For this review, take the finished solid that the model builds, in its own axes (mm). Coordinates: 2 decimals unless noted, no trailing zeros. Loops run counter-clockwise (first coordinate to the right, second up) from the corner with the lowest first, then second, coordinate; pieces in that order, holes last.
1. Take a section at A-A, the plane y = 130. State the section outline as (x, z) points, then the cut area to 3 significant figures.
2. Take a section at C-C, the plane x = -64. State the section outline as (y, z) points, then the cut area to 3 significant figures.
3. To check wall thickness, follow probe 1 along X at (y, z) = (80, 0.55); probe 2 along X at (y, z) = (145.5, 1.6); probe 3 along Y at (x, z) = (-32, 0.9). State the ranges of each line that lie inside material, in increasing order.
4. Clearance check with flat-ended pins moving along their axes: P1, Ø0.6, axis at y = 243.5, z = 1, coming from the +X side; P2, Ø0.6, axis at y = 160, z = 1.5, coming from the -X side; P3, Ø1, axis at x = -69.5, z = 1.5, coming from the +Y side. State where each tip first meets the part, or that it passes through.
5. Take a section at B-B, the plane z = 0.4. Count the separate pieces of the cut face and the enclosed holes in it, then the cut area to 3 significant figures.
6. Take a section at D-D, the plane y = 170. State the section outline as (x, z) points.
```python
from build123d import *

# Parameters (mm, degrees)
F0_W     = 20
F0_H     = 93
F0_H_2   = 79
F0_H_3   = 53
F0_H_4   = 1
F0_W_2   = 15
F0_W_3   = 2
F0_H_5   = 9
F0_W_4   = 1
F0_W_5   = 6
F1_DEPTH = 0.1
F2_DEPTH = 2


# Not quite as in the source:
# - a feature names something its author has since deleted; it is built from what else it names


with BuildPart() as f1:
    # F0 (on Top) → F1 (new body)
    with BuildSketch(Plane.XY):
        Polygon((-134.4656153619, 144.6975417137), (-143.4656153619, 144.6975417137), (-143.4656153619, 104.6975417137), (-143.4656153619, 95.6975417137), (-143.4656153619, 64.6975417137), (-143.4656153619, 60.6975417137), (-123.4656153619, 60.6975417137), (-123.4656153619, 164.6975417137), (-134.4656153619, 153.6975417137), align=None)
        Polygon((-123.4656153619, 6.6975417137), (-123.4656153619, 59.6975417137), (-143.4656153619, 59.6975417137), (-143.4656153619, 55.6975417137), (-143.4656153619, 15.6975417137), (-134.4656153619, 15.6975417137), (-134.4656153619, 6.6975417137), align=None)
        with Locations((-112.4656153619, 53.1975417137)):
            Rectangle(F0_W, F0_H)
        Polygon((-102.4656153619, 185.6975417137), (-122.4656153619, 165.6975417137), (-122.4656153619, 100.6975417137), (-102.4656153619, 100.6975417137), align=None)
        Polygon((-81.4656153619, 140.6975417137), (-81.4656153619, 206.6975417137), (-101.4656153619, 186.6975417137), (-101.4656153619, 140.6975417137), align=None)
        with Locations((-91.4656153619, 100.1975417137)):
            Rectangle(F0_W, F0_H_2)
        with Locations((-91.4656153619, 33.1975417137)):
            Rectangle(F0_W, F0_H_3)
        Polygon((-60.4656153619, 100.6975417137), (-60.4656153619, 227.6975417137), (-80.4656153619, 207.6975417137), (-80.4656153619, 100.6975417137), align=None)
        with Locations((-70.4656153619, 53.1975417137)):
            Rectangle(F0_W, F0_H)
        Polygon((-41.4656153619, 237.6975417137), (-41.4656153619, 246.6975417137), (-59.4656153619, 228.6975417137), (-59.4656153619, 140.6975417137), (-39.4656153619, 140.6975417137), (-39.4656153619, 237.6975417137), align=None)
        with Locations((-49.4656153619, 100.1975417137)):
            Rectangle(F0_W, F0_H_2)
        with Locations((-49.4656153619, 33.1975417137)):
            Rectangle(F0_W, F0_H_3)
        with Locations((-133.4656153619, 60.1975417137)):
            Rectangle(F0_W, F0_H_4)
        Polygon((-122.4656153619, 165.6975417137), (-123.4656153619, 164.6975417137), (-123.4656153619, 60.6975417137), (-123.4656153619, 59.6975417137), (-123.4656153619, 6.6975417137), (-122.4656153619, 6.6975417137), (-122.4656153619, 99.6975417137), (-122.4656153619, 100.6975417137), align=None)
        with Locations((-112.4656153619, 100.1975417137)):
            Rectangle(F0_W, F0_H_4)
        Polygon((-101.4656153619, 186.6975417137), (-102.4656153619, 185.6975417137), (-102.4656153619, 100.6975417137), (-102.4656153619, 99.6975417137), (-102.4656153619, 6.6975417137), (-101.4656153619, 6.6975417137), (-101.4656153619, 59.6975417137), (-101.4656153619, 60.6975417137), (-101.4656153619, 139.6975417137), (-101.4656153619, 140.6975417137), align=None)
        with Locations((-91.4656153619, 140.1975417137)):
            Rectangle(F0_W, F0_H_4)
        Polygon((-80.4656153619, 100.6975417137), (-80.4656153619, 207.6975417137), (-81.4656153619, 206.6975417137), (-81.4656153619, 140.6975417137), (-81.4656153619, 139.6975417137), (-81.4656153619, 60.6975417137), (-81.4656153619, 59.6975417137), (-81.4656153619, 6.6975417137), (-80.4656153619, 6.6975417137), (-80.4656153619, 99.6975417137), align=None)
        with Locations((-70.4656153619, 100.1975417137)):
            Rectangle(F0_W, F0_H_4)
        Polygon((-59.4656153619, 140.6975417137), (-59.4656153619, 228.6975417137), (-60.4656153619, 227.6975417137), (-60.4656153619, 100.6975417137), (-60.4656153619, 99.6975417137), (-60.4656153619, 6.6975417137), (-59.4656153619, 6.6975417137), (-59.4656153619, 59.6975417137), (-59.4656153619, 60.6975417137), (-59.4656153619, 139.6975417137), align=None)
        with Locations((-49.4656153619, 60.1975417137)):
            Rectangle(F0_W, F0_H_4)
        with Locations((-49.4656153619, 140.1975417137)):
            Rectangle(F0_W, F0_H_4)
        with Locations((-91.4656153619, 60.1975417137)):
            Rectangle(F0_W, F0_H_4)
        Polygon((-38.4656153619, 237.6975417137), (-39.4656153619, 237.6975417137), (-39.4656153619, 140.6975417137), (-39.4656153619, 139.6975417137), (-39.4656153619, 60.6975417137), (-39.4656153619, 59.6975417137), (-39.4656153619, 6.6975417137), (-38.4656153619, 6.6975417137), (-38.4656153619, 99.6975417137), (-38.4656153619, 100.6975417137), align=None)
        Polygon((-23.4656153619, 99.6975417137), (-38.4656153619, 99.6975417137), (-38.4656153619, 6.6975417137), (-32.4656153619, 6.6975417137), (-32.4656153619, 15.6975417137), (-23.4656153619, 15.6975417137), align=None)
        Polygon((-32.4656153619, 237.6975417137), (-38.4656153619, 237.6975417137), (-38.4656153619, 100.6975417137), (-23.4656153619, 100.6975417137), (-23.4656153619, 144.6975417137), (-32.4656153619, 144.6975417137), (-32.4656153619, 153.6975417137), (-23.4656153619, 153.6975417137), (-23.4656153619, 237.6975417137), align=None)
        with Locations((-30.9656153619, 100.1975417137)):
            Rectangle(F0_W_2, F0_H_4)
        with Locations((-40.4656153619, 242.1975417137)):
            Rectangle(F0_W_3, F0_H_5)
        with Locations((-38.9656153619, 242.1975417137)):
            Rectangle(F0_W_4, F0_H_5)
        with Locations((-35.4656153619, 242.1975417137)):
            Rectangle(F0_W_5, F0_H_5)
    extrude(amount=-F1_DEPTH)

    # F0 (on Top) → F2 (join)
    with BuildSketch(Plane.XY):
        Polygon((-134.4656153619, 144.6975417137), (-143.4656153619, 144.6975417137), (-143.4656153619, 104.6975417137), (-143.4656153619, 95.6975417137), (-143.4656153619, 64.6975417137), (-143.4656153619, 60.6975417137), (-123.4656153619, 60.6975417137), (-123.4656153619, 164.6975417137), (-134.4656153619, 153.6975417137), align=None)
        Polygon((-123.4656153619, 6.6975417137), (-123.4656153619, 59.6975417137), (-143.4656153619, 59.6975417137), (-143.4656153619, 55.6975417137), (-143.4656153619, 15.6975417137), (-134.4656153619, 15.6975417137), (-134.4656153619, 6.6975417137), align=None)
        with Locations((-112.4656153619, 53.1975417137)):
            Rectangle(F0_W, F0_H)
        Polygon((-102.4656153619, 185.6975417137), (-122.4656153619, 165.6975417137), (-122.4656153619, 100.6975417137), (-102.4656153619, 100.6975417137), align=None)
        Polygon((-81.4656153619, 140.6975417137), (-81.4656153619, 206.6975417137), (-101.4656153619, 186.6975417137), (-101.4656153619, 140.6975417137), align=None)
        with Locations((-91.4656153619, 100.1975417137)):
            Rectangle(F0_W, F0_H_2)
        with Locations((-91.4656153619, 33.1975417137)):
            Rectangle(F0_W, F0_H_3)
        with Locations((-70.4656153619, 53.1975417137)):
            Rectangle(F0_W, F0_H)
        Polygon((-60.4656153619, 100.6975417137), (-60.4656153619, 227.6975417137), (-80.4656153619, 207.6975417137), (-80.4656153619, 100.6975417137), align=None)
        Polygon((-41.4656153619, 237.6975417137), (-41.4656153619, 246.6975417137), (-59.4656153619, 228.6975417137), (-59.4656153619, 140.6975417137), (-39.4656153619, 140.6975417137), (-39.4656153619, 237.6975417137), align=None)
        with Locations((-49.4656153619, 100.1975417137)):
            Rectangle(F0_W, F0_H_2)
        with Locations((-49.4656153619, 33.1975417137)):
            Rectangle(F0_W, F0_H_3)
        Polygon((-23.4656153619, 99.6975417137), (-38.4656153619, 99.6975417137), (-38.4656153619, 6.6975417137), (-32.4656153619, 6.6975417137), (-32.4656153619, 15.6975417137), (-23.4656153619, 15.6975417137), align=None)
        Polygon((-32.4656153619, 237.6975417137), (-38.4656153619, 237.6975417137), (-38.4656153619, 100.6975417137), (-23.4656153619, 100.6975417137), (-23.4656153619, 144.6975417137), (-32.4656153619, 144.6975417137), (-32.4656153619, 153.6975417137), (-23.4656153619, 153.6975417137), (-23.4656153619, 237.6975417137), align=None)
        with Locations((-40.4656153619, 242.1975417137)):
            Rectangle(F0_W_3, F0_H_5)
        with Locations((-35.4656153619, 242.1975417137)):
            Rectangle(F0_W_5, F0_H_5)
    extrude(amount=F2_DEPTH)


solid = f1.part
```
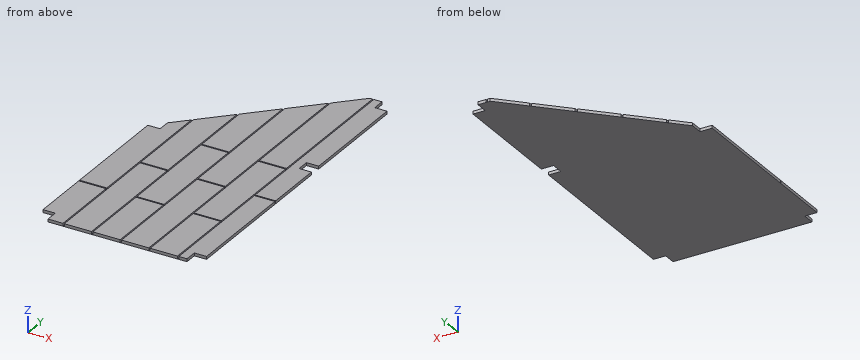
Results list:
1. outline: (-143.47, -0.1) - (-23.47, -0.1) - (-23.47, 2) - (-38.47, 2) - (-38.47, 0) - (-39.47, 0) - (-39.47, 2) - (-59.47, 2) - (-59.47, 0) - (-60.47, 0) - (-60.47, 2) - (-80.47, 2) - (-80.47, 0) - (-81.47, 0) - (-81.47, 2) - (-101.47, 2) - (-101.47, 0) - (-102.47, 0) - (-102.47, 2) - (-122.47, 2) - (-122.47, 0) - (-123.47, 0) - (-123.47, 2) - (-143.47, 2) - close
1. area: 242 mm2
2. outline: (6.7, -0.1) - (224.16, -0.1) - (224.16, 2) - (100.7, 2) - (100.7, 0) - (99.7, 0) - (99.7, 2) - (6.7, 2) - close
2. area: 455 mm2
3. probe 1: x = -143.47 to -123.47, -122.47 to -102.47, -101.47 to -81.47, -80.47 to -60.47, -59.47 to -39.47, -38.47 to -23.47
3. probe 2: x = -134.47 to -123.47, -122.47 to -102.47, -101.47 to -81.47, -80.47 to -60.47, -59.47 to -39.47, -38.47 to -32.47
3. probe 3: y = 15.7 to 99.7, 100.7 to 144.7, 153.7 to 237.7
4. P1: stops at x = -32.47
4. P2: stops at x = -128.46
4. P3: stops at y = 219.16
5. separate pieces: 14
5. enclosed holes: 0
5. area: 22,100 mm2
6. outline: (-118.16, -0.1) - (-23.47, -0.1) - (-23.47, 2) - (-38.47, 2) - (-38.47, 0) - (-39.47, 0) - (-39.47, 2) - (-59.47, 2) - (-59.47, 0) - (-60.47, 0) - (-60.47, 2) - (-80.47, 2) - (-80.47, 0) - (-81.47, 0) - (-81.47, 2) - (-101.47, 2) - (-101.47, 0) - (-102.47, 0) - (-102.47, 2) - (-118.16, 2) - close
